Geometry check sheet. Reference: the model listing, model coordinates, mm. Give positions to 0.01 mm unless a question says otherwise; leave off trailing zeros. Order: outer loops, then holes, each group sorted by start corner. A loop starts at its lowest first (then second) coordinate and runs counter-clockwise, first axis right, second up.
Autodesk Inventor part; units mm, degrees
ref_plane "YZ Plane" through (0, 0, 0) normal (1, 0, 0) x (0, 1, 0)
ref_plane "XZ Plane" through (0, 0, 0) normal (0, 1, 0) x (-1, 0, 0)
ref_plane "XY Plane" through (0, 0, 0) normal (0, 0, 1) x (1, 0, 0)
ref_plane "Work Plane1" through (0, 0, 0) normal (0, 0, 1) x (1, 0, 0)
sketch "Sketch1" plane through (0, 0, 0) normal (0, 0, 1) x (1, 0, 0)
  circle A0 centre (29.5896, 9.9505) radius 2
  circle A1 centre (32.2876, 59.8777) radius 2.5
  line L0 (29.5896, 9.9505) -> (29.5896, -30.0495)
  line L1 (29.5896, -30.0495) -> (79.5896, -30.0495)
  line L2 (79.5896, -30.0495) -> (79.5896, 89.9505)
  line L3 (79.5896, 89.9505) -> (-20.4104, 89.9505)
  line L4 (-20.4104, 89.9505) -> (79.5896, 89.9505)
  line L5 (79.5896, 89.9505) -> (79.5896, -30.0495)
  line L6 (79.5896, -30.0495) -> (-20.4104, -30.0495)
  line L7 (-20.4104, -30.0495) -> (-20.4104, 89.9505)
  circle A2 centre (16.7876, 75.3777) radius 1.6
  circle A3 centre (47.7876, 75.3777) radius 1.6
  circle A4 centre (47.7876, 44.3777) radius 1.6
  circle A5 centre (16.7876, 44.3777) radius 1.6
  line L8 (-20.4104, 89.9505) -> (-10.4104, 89.9505)
  line L9 (-10.4104, 89.9505) -> (-10.4104, 69.9505)
  line L10 (-10.4104, 69.9505) -> (-10.4104, 49.9505)
  line L11 (-10.4104, 49.9505) -> (-10.4104, 29.9505)
  line L12 (-10.4104, 29.9505) -> (-10.4104, 9.9505)
  line L13 (-10.4104, 9.9505) -> (-10.4104, -10.0495)
  line L14 (79.5896, 89.9505) -> (69.5896, 89.9505)
  line L15 (69.5896, 89.9505) -> (69.5896, 69.9505)
  line L16 (69.5896, 69.9505) -> (69.5896, 49.9505)
  line L17 (69.5896, 49.9505) -> (69.5896, 29.9505)
  line L18 (69.5896, 29.9505) -> (69.5896, 9.9505)
  line L19 (69.5896, 9.9505) -> (69.5896, -10.0495)
  circle A6 centre (-10.4104, 69.9505) radius 4
  circle A7 centre (-10.4104, 49.9505) radius 4
  circle A8 centre (-10.4104, 29.9505) radius 4
  circle A9 centre (-10.4104, 9.9505) radius 4
  circle A10 centre (-10.4104, -10.0495) radius 4
  circle A11 centre (69.5896, 69.9505) radius 4
  circle A12 centre (69.5896, 49.9505) radius 4
  circle A13 centre (69.5896, 29.9505) radius 4
  circle A14 centre (69.5896, 9.9505) radius 4
  circle A15 centre (69.5896, -10.0495) radius 4
  dimension "d0" = 4
  dimension "d1" = 5
  dimension "d2" = 40
  dimension "d3" = 50
  dimension "d4" = 120
  dimension "d5" = 100
  dimension "d6" = 3.2
  dimension "d7" = 3.2
  dimension "d8" = 3.2
  dimension "d9" = 3.2
  dimension "d10" = 10
  dimension "d11" = 20
  dimension "d12" = 20
  dimension "d13" = 20
  dimension "d14" = 20
  dimension "d15" = 20
  dimension "d16" = 10
  dimension "d17" = 20
  dimension "d18" = 20
  dimension "d19" = 20
  dimension "d20" = 20
  dimension "d21" = 20
  dimension "d22" = 8
  dimension "d23" = 8
  dimension "d24" = 8
  dimension "d25" = 8
  dimension "d26" = 8
  dimension "d27" = 8
  dimension "d28" = 8
  dimension "d29" = 8
  dimension "d30" = 8
  dimension "d31" = 8
extrude "Extrusion1" add sketch "Sketch1" along normal blind 6
properties part number "motor_gear_holder"
Item 1: Sectioned sample at A-A (z = 3.35). Give the number of separate pieces and of enclosed holes in the cut face, and give its area (3 significant figures).
Reported:
separate pieces: 1
enclosed holes: 16
area: 11,400 mm2
Item 2: Sectioned sample at B-B (x = 67). Enter the section's corners in (y, z), and give its area (3 significant figures).
Reported:
outline: (-30.05, 0) - (-13.1, 0) - (-13.1, 6) - (-30.05, 6) - close; (-7, 0) - (6.9, 0) - (6.9, 6) - (-7, 6) - close; (13, 0) - (26.9, 0) - (26.9, 6) - (13, 6) - close; (33, 0) - (46.9, 0) - (46.9, 6) - (33, 6) - close; (53, 0) - (66.9, 0) - (66.9, 6) - (53, 6) - close; (73, 0) - (89.95, 0) - (89.95, 6) - (73, 6) - close
area: 537 mm2
Item 3: Scan lines: L1, parallel to Y at x = 47.5, z = 4.05; L2, parallel to X at y = 30, z = 0.95; L3, parallel to Y at x = -10, z = 2.4. Record each from-to range of solid material in increasing order.
Reported:
L1: y = -30.05 to 42.8, 45.95 to 73.8, 76.95 to 89.95
L2: x = -20.41 to -14.41, -6.41 to 65.59, 73.59 to 79.59
L3: y = -30.05 to -14.03, -6.07 to 5.97, 13.93 to 25.97, 33.93 to 45.97, 53.93 to 65.97, 73.93 to 89.95
Item 4: Draft check along Y on faces 1 (the flat face through (29, 31, 0)), 2 (the cylindrical face through (18.314, 74.897, 2.958)), 3 (the flat face through (30, -30.05, 3)). Enter one of: released by +Y, released by -Y, zero draft, split by the parting line, or undercut.
Reported:
face 1: zero draft
face 2: undercut
face 3: released by -Y
